Build history of the part. All positions in model axes, mm. Face numbers are marked on the shaded views. A direction names the side the tool comes from. Coordinates: 2 decimals unless noted, no trailing zeros. Loops run counter-clockwise (first coordinate to the right, second up) from the corner with the lowest first, then second, coordinate; pieces in that order, holes last.
(1) Slice it at B-B (z = 10). Give the cut face in (x, y), and give its area (3 significant figures).
(2) Flat gauge pins, fed straight in: P1, Ø3, axis at x = 6.5, z = -10, coming from the +Y side; P2, Ø4, axis at x = 5, z = 35.5, coming from the +Y side; P3, Ø1.5, axis at y = -9.5, z = 29.5, coming from the +X side. Where does each tip first touch, or does it go through?
(3) Slice it at D-D (y = -9.5). Give the cut face in (x, z).
(4) Two-plate mould, pull along Z, no slides. Class the marked faces 1, 2, 3 and 4: pulls with the +Z half, pulls with the -Z half, needs draft (parallel to the pull), parting line crosses it, or undercut.
(5) Tool access for the marked faces 5, 6, 7 and 8: list every direction of +Z, -Z, +X, -X, +Y, -Y with a clear straight run to the whole face (end or side of a thin tool).
(6) Wall check: L1, parallel to X at y = -9, z = 31.5; L2, parallel to Y at x = 4.25, z = 13.5; L3, parallel to Y at x = 6.5, z = 40. Give the ranges that are in metal, low to high.
(7) Slice it at A-A (x = 8.25). Give the number of separate pieces and of enclosed holes in the cut face, and give its area (3 significant figures).
(8) Slice it at C-C (x = 0.75). Give the cut face in (y, z).
from build123d import *

# Parameters (mm, degrees)
F1_DEPTH = 10
F2_R     = 1.75
F3_DEPTH = 25
F4_R     = 1.75
F5_DEPTH = 6.5
F6_W     = 7.5
F6_H     = 5
F7_DEPTH = 52.6


with BuildPart() as f1:
    # F0 (on Right) → F1 (new body)
    with BuildSketch(Plane.YZ):
        Polygon((-20, 49.6487663492), (-20, 0), (0, 0), (0, -20), (4, -20), (4, 0), (3.6312381011, 0.9295238899), (1.4186667076, 6.5066672293), (1.0499048087, 7.4361911193), (-18.8632377328, 57.6304811742), (-19.2319996317, 58.5600050641), (-21.4445710252, 64.1371484036), (-21.8133329241, 65.0666722935), (-25.5314284837, 63.5916246978), align=None)
        Polygon((-16, 4), (-16, 39.5661206894), (-1.8901633999, 4), align=None, mode=Mode.SUBTRACT)
        Polygon((-18.0952373645, 66.5417198892), (-21.8133329241, 65.0666722935), (-21.4445710252, 64.1371484036), (-19.5855232454, 64.8746722014), (-17.3729518519, 59.297528862), (-19.2319996317, 58.5600050641), (-18.8632377328, 57.6304811742), (-15.1451421732, 59.1055287699), align=None)
        Polygon((3.6312381011, 0.9295238899), (4, 0), (7.7180955596, 1.4750475957), (4.7680003683, 8.9112387149), (1.0499048087, 7.4361911193), (1.4186667076, 6.5066672293), (3.2777144874, 7.2441910272), (5.4902858809, 1.6670476877), align=None)
    extrude(amount=F1_DEPTH)

    # F2 (on face) → F3 (cut)
    with BuildSketch(Plane(origin=(0, 7.1741542073, 2.8461395746), x_dir=(-1, 0, 0), z_dir=(0, 0.9295238899, 0.3687618989))):
        with Locations((-5, 64.5249524043)):
            Circle(F2_R)
    extrude(amount=-F3_DEPTH, mode=Mode.SUBTRACT)

    # F4 (on face) → F5 (cut)
    with BuildSketch(Plane(origin=(0, 7.1741542073, 2.8461395746), x_dir=(-1, 0, 0), z_dir=(0, 0.9295238899, 0.3687618989))):
        with Locations((-5, 2.5249524043)):
            Circle(F4_R)
    extrude(amount=-F5_DEPTH, mode=Mode.SUBTRACT)

    # F6 (on face) → F7 (cut)
    with BuildSketch(Plane(origin=(0, 0, 0), x_dir=(1, 0, 0), z_dir=(0, 0, -1))):
        with Locations((6.25, 10)):
            Rectangle(F6_W, F6_H)
    extrude(amount=-F7_DEPTH, mode=Mode.SUBTRACT)


solid = f1.part
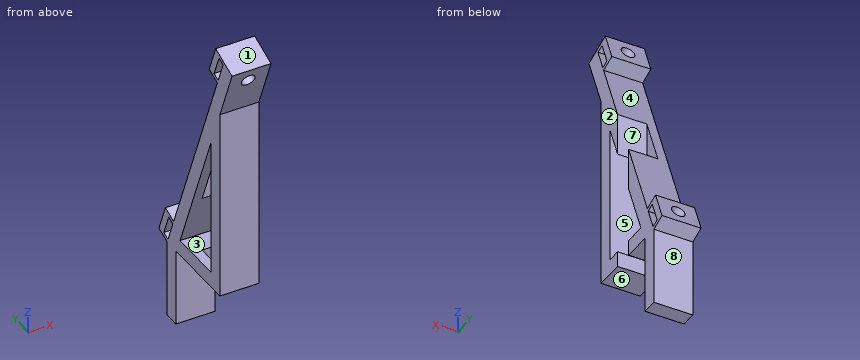
Response values:
1. outline: (0, -20) - (10, -20) - (10, -16) - (0, -16) - close; (0, -4.27) - (10, -4.27) - (10, 0.03) - (0, 0.03) - close
1. area: 83.0 mm2
2. P1: stops at y = 4
2. P2: stops at y = -12.5
2. P3: stops at x = 2.5
3. outline: (0, 0) - (2.5, 0) - (2.5, 4) - (0, 4) - close; (0, 23.18) - (2.5, 23.18) - (2.5, 34.03) - (0, 34.03) - close
4. face 1: pulls with the +Z half
4. face 2: needs draft
4. face 3: undercut
4. face 4: undercut
5. face 5: +X, -X
5. face 6: -Z, +X, -X, -Y
5. face 7: +Z, -Z, +X, +Y
5. face 8: -Z, +X, -X, +Y
6. L1: x = 0 to 2.5
6. L2: y = -20 to -16, -5.66 to -1.36
6. L3: y = -20 to -12.5
7. separate pieces: 2
7. enclosed holes: 2
7. area: 561 mm2
8. outline: (-25.53, 63.59) - (-20, 49.65) - (-20, 0) - (0, 0) - (0, -20) - (4, -20) - (4, 0) - (7.72, 1.48) - (4.77, 8.91) - (1.05, 7.44) - (-18.86, 57.63) - (-15.15, 59.11) - (-18.1, 66.54) - close; hole (-21.44, 64.14) - (-19.23, 58.56) - (-17.37, 59.3) - (-19.59, 64.87) - close; hole (-16, 4) - (-1.89, 4) - (-16, 39.57) - close; hole (1.42, 6.51) - (3.63, 0.93) - (5.49, 1.67) - (3.28, 7.24) - close
